from build123d import *

# Parameters (mm, degrees)
EXTRUDE_1_DEPTH     = 20
SKETCH_2_R          = 5
CUT_EXTRUDE_1_DEPTH = 757.029761319
SKETCH_3_R          = 5.15
CUT_EXTRUDE_2_DEPTH = 20
CUT_EXTRUDE_START   = -20
SKETCH_4_R          = 5.15
CUT_EXTRUDE_3_DEPTH = 20
SKETCH_5_R          = 1.25
CUT_EXTRUDE_4_DEPTH = 10


with BuildPart() as part:
    # 草图1 → 凸台-拉伸1 (new body)
    with BuildSketch(Plane.XY):
        Polygon((0, 0), (466, 0), (466, -595), (151, -595), (151, -225), (0, -225), align=None)
    extrude(amount=-EXTRUDE_1_DEPTH)

    # 草图2 → 切除-拉伸1 (cut, through all)
    with BuildSketch(Plane.XY):
        with Locations((43.2, -32)):
            Circle(SKETCH_2_R)
        with Locations((459, -30)):
            Circle(SKETCH_2_R)
        with Locations((459, -105)):
            Circle(SKETCH_2_R)
        with Locations((7.2, -107)):
            Circle(SKETCH_2_R)
        with BuildLine():
            Line((218.5, -595), (218.5, -525))
            ThreePointArc((218.5, -525), (227.286796564, -503.786796564), (248.5, -495))
            Line((248.5, -495), (368.5, -495))
            ThreePointArc((368.5, -495), (389.713203436, -503.786796564), (398.5, -525))
            Line((398.5, -525), (398.5, -595))
            Line((398.5, -595), (218.5, -595))
        make_face()
    extrude(amount=-CUT_EXTRUDE_1_DEPTH, mode=Mode.SUBTRACT)

    # 草图3 → 切除-拉伸2 (cut)
    with BuildSketch(Plane.ZY):
        with Locations((-10, -155)):
            Circle(SKETCH_3_R)
        with Locations((-10, -205)):
            Circle(SKETCH_3_R)
    extrude(amount=-CUT_EXTRUDE_2_DEPTH, mode=Mode.SUBTRACT)

    # 草图4 → 切除-拉伸3 (cut)
    with BuildSketch(Plane(origin=(466, 0, 0), x_dir=(0, 0, -1), z_dir=(1, 0, 0)).offset(CUT_EXTRUDE_START)):
        with Locations(Location((10, -155, 0), (0, 0, 180))):
            Circle(SKETCH_4_R)
        with Locations(Location((10, -205, 0), (0, 0, 180))):
            Circle(SKETCH_4_R)
    extrude(amount=CUT_EXTRUDE_3_DEPTH, mode=Mode.SUBTRACT)

    # 草图5 → 切除-拉伸4 (cut)
    with BuildSketch(Plane(origin=(0, 0, 0), x_dir=(1, 0, 0), z_dir=(0, 1, 0))):
        with Locations(Location((32, 15, 0), (0, 0, 270))):
            Circle(SKETCH_5_R)
        with Locations(Location((32, 5, 0), (0, 0, 270))):
            Circle(SKETCH_5_R)
        with Locations(Location((422, 15, 0), (0, 0, 270))):
            Circle(SKETCH_5_R)
        with Locations(Location((422, 5, 0), (0, 0, 270))):
            Circle(SKETCH_5_R)
    extrude(amount=-CUT_EXTRUDE_4_DEPTH, mode=Mode.SUBTRACT)


solid = part.part
Read the model definition and answer for the solid it produces. Units are mm, in the model's axes. A direction names the side the tool comes from. Round coordinates to 2 decimals unless told otherwise and drop trailing zeros. Write each loop counter-clockwise with the first axis right and the second up, starting at its lowest first coordinate (ties: lowest second). Pieces come first, ordered by that corner, then holes. Notation, with made-up numbers: (32, 16) - (51, 16) arc R13 cw to (51, 31) - close; hole circle Ø4 at (3.25, 14). An arc over 180 degrees is marked (long way). One line per question, with ' | ' between items. Start each with the question number.
1. Section B-B (x = 377) is taken. Determine the outline of the cut face in (y, z).
2. For faces 1 (the face through (77, -225, -10)), 2 (the face through (466, -293, -10)), 3 (the face through (218.5, -560, -10)), determine the directions among +Z, -Z, +X, -X, +Y, -Y from which every point of the face is accessible in a straight line to the end or side of a thin tool.
3. For a pull along X with two mould halves and no side action, classify faces 4 (the face through (227.055, -504.021, -9.86)), 5 (the face through (230, 0, -10)), 6 (the face through (398.5, -560, -10)), 7 (the face through (0, -114, -10)) as +X half, -X half, draft (parallel to the pull), parting line (faces both ways), or undercut.
4. Find the intervals of material crossed by probe 1 along X at (y, z) = (-6.25, -15); probe 2 along Y at (x, z) = (16, -10); probe 3 along Y at (x, z) = (452.75, -10), in increasing order. Write a range as [from, to].
5. Section A-A (y = -278.5) is taken. Determine the outline of the cut face in (x, z), and give its area (3 significant figures).
6. Each of these flat-tipped pins is pushed along its axis until it touches: pin 1 (1 mm diameter, centred on y = -378.5, z = -13, fed in from -X); pin 2 (0.8 mm diameter, centred on x = 32, z = -5, fed in from +Y); pin 3 (9.5 mm diameter, centred on y = -205, z = -10, fed in from +X); pin 4 (8 mm diameter, centred on x = 459, y = -105, fed in from +Z). Where does it stop, or does it pass through?
Filled in:
1) outline: (-496.23, -20) - (0, -20) - (0, 0) - (-496.23, 0) - close
2) face 1: +Z, -Z, -X, -Y | face 2: +Z, -Z, +X, +Y, -Y | face 3: +Z, -Z, -Y
3) face 4: undercut | face 5: draft | face 6: undercut | face 7: -X half
4) probe 1: [0, 30.75], [33.25, 420.75], [423.25, 466] | probe 2: [-225, -210.15], [-199.85, -160.15], [-149.85, 0] | probe 3: [-595, -210.15], [-199.85, -160.15], [-149.85, 0]
5) outline: (151, -20) - (466, -20) - (466, 0) - (151, 0) - close | area: 6,300 mm²
6) pin 1: x = 151 | pin 2: y = -10 | pin 3: x = 446 | pin 4: through
